Autodesk Inventor part; units mm, degrees
ref_plane "YZ Plane" through (0, 0, 0) normal (1, 0, 0) x (0, 1, 0)
ref_plane "XZ Plane" through (0, 0, 0) normal (0, 1, 0) x (-1, 0, 0)
ref_plane "XY Plane" through (0, 0, 0) normal (0, 0, 1) x (1, 0, 0)
sketch "Sketch1" plane through (0, 0, 0) normal (0, 0, 1) x (1, 0, 0)
  line L0 (0, 0) -> (-40, 0)
  line L1 (-40, 0) -> (-40, 50)
  line L2 (-40, 50) -> (0, 50)
  line L3 (0, 50) -> (0, 0)
  dimension "d0" = 50
  dimension "d1" = 40
extrude "Extrusion1" add sketch "Sketch1" along normal blind 40
sketch "Sketch2" plane through (-40, 50, 0) normal (0, 1, 0) x (1, 0, 0)
  line L0 (40, 0) -> (0, 0)
  line L1 (0, 0) -> (0, -40)
  line L2 (40, -40) -> (0, -40)
  line L3 (40, 0) -> (40, -40)
  line L4 (5, -5) -> (35, -5)
  line L5 (35, -5) -> (35, -35)
  line L6 (35, -35) -> (5, -35)
  line L7 (5, -35) -> (5, -5)
  dimension "d5" = 5
extrude "Extrusion2" cut sketch "Sketch2" against normal blind 30 contours L4 L5 L6 L7
sketch "Sketch3" plane through (-40, 0, 0) normal (0, -1, 0) x (1, 0, 0)
  circle A0 centre (5, 35) radius 2.5
  line L0 (5, 35) -> (7.3437, 35)
  line L1 (7.3437, 35) -> (7.3437, 32.7108)
  circle A1 centre (35, 35) radius 2.5
  circle A2 centre (5, 5) radius 2.5
  circle A3 centre (35, 5) radius 2.5
  line L2 (0, 40) -> (40, 40)
  line L3 (0, 0) -> (0, 40)
  point P0 (40, 0)
  dimension "d10" = 30
  dimension "d13" = 30
  dimension "d16" = 5
  dimension "d17" = 5
  dimension "d18" = 5
extrude "Extrusion3" cut sketch "Sketch3" against normal blind 10
sketch "Sketch4" plane through (-40, 50, 0) normal (0, 1, 0) x (1, 0, 0)
  line L0 (0, 0) -> (0, -40)
  line L1 (0, -25) -> (-10, -25)
  line L2 (-10, -25) -> (-10, -15)
  line L3 (-10, -15) -> (0, -15)
  line L4 (0, -15) -> (0, -25)
  line L5 (40, 0) -> (40, -40)
  line L6 (40, -25) -> (50, -25)
  line L7 (50, -25) -> (50, -15)
  line L8 (50, -15) -> (40, -15)
  line L9 (40, -15) -> (40, -25)
  line L10 (-23.587, -20) -> (57.8749, -20)
  line L11 (40, -40) -> (0, -40)
  line L12 (35, -5) -> (35, -35)
  line L13 (35, -35) -> (5, -35)
  line L14 (5, -35) -> (5, -5)
  line L15 (5, -5) -> (35, -5)
  line L16 (40, 0) -> (0, 0)
  line L17 (0, 0) -> (0, -40)
  line L18 (40, -40) -> (0, -40)
  line L19 (40, 0) -> (40, -40)
  circle A0 centre (-5, -20) radius 2.75
  circle A1 centre (45, -20) radius 2.75
  point P0 (0, -20)
  point P1 (0, -20)
  point P2 (-5, -15)
  point P3 (45, -15)
  dimension "d21" = 10
  dimension "d22" = 10
  dimension "d23" = 10
  dimension "d26" = 5.5
  dimension "d27" = 5.5
extrude "Extrusion4" add sketch "Sketch4" against normal blind 10 contours L0 L10 A0 L2 L3 | L0 L1 L2 L10 A0 | L8 L7 L10 A1 L5 | L10 A1 L7 L6 L5
properties part number "battery5V_box"
The listing builds one solid part. Answer for the finished solid, in the listing's coordinates (mm). A direction names the side the tool comes from. Coordinates: 2 decimals unless noted, no trailing zeros. Write each loop counter-clockwise with the first axis right and the second up, starting at its lowest first coordinate (ties: lowest second). Pieces come first, ordered by that corner, then holes. Notation, with made-up numbers: (-22, 26) - (21, 26) arc R13 ccw to (21, 39) - close; hole circle Ø2 at (63.5, 25). An arc over 180 degrees is marked (long way). Return JSON: item names as keys, results as strings. Group by question number.
Q1. Which of the six approach directions +Z, -Z, +X, -X, +Y, -Y give full straight-line access (tool end or side, diameter ignored) to faces 4 (the flat face through (5, 45, 15)), 5 (the flat face through (7.2, 40, 22.2)), 6 (the cylindrical face through (-2.615, 4.93, 5.751)), 7 (the flat face through (-35, 35, 20)), 8 (the flat face through (5, 45, 25))?
Q2. The part is cut by section D-D on x = -9.5. Write down the section's boundary in (y, z).
Q3. The part is cut by section B-B on x = 5. Write down the section's boundary in (y, z).
Q4. The part is cut by section C-C on z = 18. Write down the section's boundary in (x, y).
Q5. The part is cut by section A-A on y = 44. Write down the section's boundary in (x, z), and give its area (3 significant figures).
Q6. Find the intervals of material crossed by line 1 along Z through (x, y) = (-35, 7); line 2 along Z through (x, y) = (-34.5, 38.5); line 3 along X through (y, z) = (43.75, 20), in increasing order. Write a range as [from, to].
Q7. For a pull along X with two mould halves and no side action, classify faces 1 (the flat face through (-45, 45, 25)), 2 (the flat face through (-5, 10, 35)), 3 (the cylindrical face through (-32.69, 4.93, 4.04)) as +X half, -X half, draft (parallel to the pull), parting line (faces both ways), or undercut.
Q8. Flat-ended cylindrical pins translate along their axes: pin 1 Ø11 at (x, y) = (6.5, 43) entering from +Z; pin 2 Ø4.5 at (x, z) = (-35, 35) entering from -Y; pin 3 Ø8 at (x, z) = (4.5, 21.5) entering from -Y. Find the tip coordinate at first contact, or state that the pin passes through.
Evaluation:
{
 "1": {"face 4": "-Z, +X, +Y, -Y", "face 5": "+Z, -Z, +X, -Y", "face 6": "-Y", "face 7": "+Y", "face 8": "+Z, +X, +Y, -Y"},
 "2": {"outline": "(0, 0) - (50, 0) - (50, 5) - (20, 5) - (20, 35) - (50, 35) - (50, 40) - (0, 40) - close"},
 "3": {"outline": "(40, 15) - (50, 15) - (50, 17.25) - (40, 17.25) - close; (40, 22.75) - (50, 22.75) - (50, 25) - (40, 25) - close"},
 "4": {"outline": "(-50, 40) - (-46.89, 40) - (-46.89, 50) - (-50, 50) - close; (-43.11, 40) - (-40, 40) - (-40, 0) - (0, 0) - (0, 40) - (3.11, 40) - (3.11, 50) - (-5, 50) - (-5, 20) - (-35, 20) - (-35, 50) - (-43.11, 50) - close; (6.89, 40) - (10, 40) - (10, 50) - (6.89, 50) - close"},
 "5": {"outline": "(-50, 15) - (-40, 15) - (-40, 0) - (0, 0) - (0, 15) - (10, 15) - (10, 25) - (0, 25) - (0, 40) - (-40, 40) - (-40, 25) - (-50, 25) - close; hole circle Ø5.5 at (-45, 20); hole (-35, 5) - (-5, 5) - (-5, 35) - (-35, 35) - close; hole circle Ø5.5 at (5, 20)", "area": "852 mm2"},
 "6": {"line 1": "z = [0, 2.5], [7.5, 32.5], [37.5, 40]", "line 2": "z = [0, 5], [35, 40]", "line 3": "x = [-50, -47.75], [-42.25, -35], [-5, 2.25], [7.75, 10]"},
 "7": {"face 1": "draft", "face 2": "undercut", "face 3": "undercut"},
 "8": {"pin 1": "stops at z = 25", "pin 2": "stops at y = 10", "pin 3": "stops at y = 40"}
}
